Geometry check sheet. Reference: the model listing, model coordinates, mm. A direction names the side the tool comes from. Coordinates: 2 decimals unless noted, no trailing zeros. Write each loop counter-clockwise with the first axis right and the second up, starting at its lowest first coordinate (ties: lowest second). Pieces come first, ordered by that corner, then holes. Notation, with made-up numbers: M 52,75.25 L 84,75.25 A10 cw 84,82.25 Z; hole C 17,35 d5. An arc over 180 degrees is marked long. Put each result on its own line as item: value. Start each with the question number.
1) Cross-section at D-D on y = 4. Record the cut outline in (x, z).
2) Cross-section at C-C on z = 72. Record the cut outline in (x, y), plus the area to 3 significant figures.
3) Cross-section at A-A on x = -23.5. Record the cut outline in (y, z).
4) Set-up check for faces 1 (the flat face through (-22, -31, 75.936)), 2 (the flat face through (-33, 64.925, 63)), 3 (the flat face through (-43.681, -31, 37)), 4 (the flat face through (-30.8, 15, 139)): record each of +Z, -Z, +X, -X, +Y, -Y from which the full face is reachable in a straight line by a thin tool's end or side.
5) Scan lines: line 1 along Y through (x, z) = (9, 53); line 2 along X through (y, z) = (-19.5, 28); line 3 along Z through (x, y) = (-33, 66). Record each from-to range of solid material in increasing order.
6) Gauge pin test, flat ends, axial feed: pin 1 (7.5 mm diameter, centred on y = 49, z = 32.5, fed in from -X); pin 2 (15.5 mm diameter, centred on x = -13, z = 114.5, fed in from +Y); pin 3 (12 mm diameter, centred on y = 22, z = 70.5, fed in from -X). Record the tip position at first contact, or that the pin passes through.
7) Cross-section at B-B on y = 39. Record the cut outline in (x, z).
from build123d import *

# Parameters (mm, degrees)
F0_W      = 75.6071731448
F0_H      = 75.7589936256
F1_DEPTH  = 25.4
F2_W      = 70.1403468847
F2_H      = 69.1941156983
F3_DEPTH  = 25.4
F4_W      = 65.8708810806
F4_H      = 64.9246573448
F5_DEPTH  = 25.4
F6_W      = 30.8003034443
F6_H      = 31.0739278793
F7_DEPTH  = 127
F8_W      = 43.6810515821
F8_H      = 75.9361535311
F9_DEPTH  = 63.5
F10_W     = 45.3466251493
F10_H     = 75.6209716201
F11_DEPTH = 63.5


with BuildPart() as f1:
    # F0 (on Top) → F1 (new body)
    with BuildSketch(Plane.XY):
        with Locations((-37.8035865724, 37.8794968128)):
            Rectangle(F0_W, F0_H)
    extrude(amount=F1_DEPTH)

    # F2 (on face) → F3 (join)
    with BuildSketch(Plane.XY.offset(25.4)):
        with Locations((-35.0701734424, 34.5970578492)):
            Rectangle(F2_W, F2_H)
    extrude(amount=F3_DEPTH)

    # F4 (on face) → F5 (join)
    with BuildSketch(Plane.XY.offset(50.8)):
        with Locations((-32.9354405403, 32.4623286724)):
            Rectangle(F4_W, F4_H)
    extrude(amount=F5_DEPTH)

    # F6 (on face) → F7 (join)
    with BuildSketch(Plane.XY.offset(76.2)):
        with Locations((-15.4001517221, 15.5369639397)):
            Rectangle(F6_W, F6_H)
    extrude(amount=F7_DEPTH)

    # F8 (on Front) → F9 (join)
    with BuildSketch(Plane.XZ):
        with Locations((-21.840525791, 37.9680767655)):
            Rectangle(F8_W, F8_H)
    extrude(amount=F9_DEPTH)

    # F10 (on Right) → F11 (join)
    with BuildSketch(Plane.YZ):
        with Locations((22.6733125746, 37.81048581)):
            Rectangle(F10_W, F10_H)
    extrude(amount=F11_DEPTH)


solid = f1.part
Answer key:
1. outline: M -75.61,0 L 63.5,0 L 63.5,75.62 L 0,75.62 L 0,203.2 L -30.8,203.2 L -30.8,76.2 L -65.87,76.2 L -65.87,50.8 L -70.14,50.8 L -70.14,25.4 L -75.61,25.4 Z
2. outline: M -65.87,0 L -43.68,0 L -43.68,-63.5 L 0,-63.5 L 0,0 L 63.5,0 L 63.5,45.35 L 0,45.35 L 0,64.92 L -65.87,64.92 Z
2. area: 9,930 mm²
3. outline: M -63.5,0 L 75.76,0 L 75.76,25.4 L 69.19,25.4 L 69.19,50.8 L 64.92,50.8 L 64.92,76.2 L 31.07,76.2 L 31.07,203.2 L 0,203.2 L 0,75.94 L -63.5,75.94 Z
4. face 1: +Z, +X, -X, -Y
4. face 2: +Z, +X, -X, +Y
4. face 3: +Z, -Z, -X, -Y
4. face 4: +Z, -X, +Y, -Y
5. line 1: y = 0 to 45.35
5. line 2: x = -43.68 to 0
5. line 3: z = 0 to 50.8
6. pin 1: stops at x = -70.14
6. pin 2: stops at y = 31.07
6. pin 3: stops at x = -65.87
7. outline: M -75.61,0 L 63.5,0 L 63.5,75.62 L 0,75.62 L 0,76.2 L -65.87,76.2 L -65.87,50.8 L -70.14,50.8 L -70.14,25.4 L -75.61,25.4 Z
